```python
from build123d import *

# Parameters (mm, degrees)
ESTRUSIONE_ESTRUSIONE1_DEPTH = 10
SCHIZZO3_W                   = 8
SCHIZZO3_H                   = 6
TAGLIO_ESTRUSIONE2_DEPTH     = 60.371710435
TAGLIO_ESTRUSIONE3_DEPTH     = 60.371710435


with BuildPart() as part:
    # Schizzo1 → Estrusione-Estrusione1 (new body)
    with BuildSketch(Plane(origin=(0, 0, 0), x_dir=(1, 0, 0), z_dir=(0, 1, 0))):
        with BuildLine():
            Line((-25, 37.416573868), (-25, 30))
            Line((-25, 30), (25, 30))
            Line((25, 30), (25, 37.416573868))
            ThreePointArc((25, 37.416573868), (45, 0), (25, -37.416573868))
            Line((25, -37.416573868), (25, -30))
            Line((25, -30), (-25, -30))
            Line((-25, -30), (-25, -37.416573868))
            ThreePointArc((-25, -37.416573868), (-45, 0), (-25, 37.416573868))
        make_face()
    extrude(amount=ESTRUSIONE_ESTRUSIONE1_DEPTH)

    # Schizzo3 → Taglio-Estrusione2 (cut, through all)
    with BuildSketch(Plane(origin=(0, 10, 0), x_dir=(1, 0, 0), z_dir=(0, 1, 0))):
        with BuildLine():
            Line((-4, -3), (-4, 3))
            ThreePointArc((-4, 3), (-5, 0), (-4, -3))
        make_face()
        Rectangle(SCHIZZO3_W, SCHIZZO3_H)
        with BuildLine():
            ThreePointArc((5, 0), (4.74341649, 1.58113883), (4, 3))
            Line((4, 3), (4, -3))
            ThreePointArc((4, -3), (4.74341649, -1.58113883), (5, 0))
        make_face()
    extrude(amount=-TAGLIO_ESTRUSIONE2_DEPTH, mode=Mode.SUBTRACT)

    # Schizzo5 → Taglio-Estrusione3 (cut, through all)
    with BuildSketch(Plane(origin=(0, 10, 0), x_dir=(1, 0, 0), z_dir=(0, 1, 0))):
        Polygon((8, -25), (8, -28.5), (8, -30), (12, -30), (12, -27), (12, -25), (13.5, -25), (13.5, -21.5), (6.5, -21.5), (6.5, -25), align=None)
        Polygon((-13.5, 21.5), (-6.5, 21.5), (-6.5, 25), (-8, 25), (-8, 28.5), (-8, 30), (-12, 30), (-12, 28.5), (-12, 25), (-13.5, 25), align=None)
        Polygon((6.5, 21.5), (13.5, 21.5), (13.5, 25), (12, 25), (12, 27), (12, 30), (8, 30), (8, 28.5), (8, 25), (6.5, 25), align=None)
        Polygon((-8, -28.5), (-8, -25), (-6.5, -25), (-6.5, -21.5), (-13.5, -21.5), (-13.5, -25), (-12, -25), (-12, -28.5), (-12, -30), (-8, -30), align=None)
    extrude(amount=-TAGLIO_ESTRUSIONE3_DEPTH, mode=Mode.SUBTRACT)


solid = part.part
```
Input: part model. Units: mm. Frame: model coordinates. A direction names the side the tool comes from. Give positions to 0.01 mm unless a question says otherwise; leave off trailing zeros. Write each loop counter-clockwise with the first axis right and the second up, starting at its lowest first coordinate (ties: lowest second). Pieces come first, ordered by that corner, then holes. Notation, with made-up numbers: (6.25, -7.75) - (26.25, -7.75) arc R22 cw to (26.25, 11.25) - close; hole circle Ø2 at (68.25, -18.75). An arc over 180 degrees is marked (long way). Write item = value, one per line. Start each with the question number.
1) Draft query along Z for faces 5 (the face through (6.5, 5, 23)), 6 (the face through (10, 5, -21.5)), 7 (the face through (-8, 5, 28)), 8 (the face through (19, 5, 30)). Return one class per face: pulls with the +Z half, pulls with the -Z half, needs draft (parallel to the pull), parting line crosses it, or undercut.
2) Pin query (flat end, axial travel): pin 1 (1.6 mm diameter, centred on x = 13, y = 4.5, fed in from -Z); pin 2 (5.5 mm diameter, centred on x = -11, y = 3.5, fed in from +Z); pin 3 (4 mm diameter, centred on y = 4.5, z = 24, fed in from -X). Return the tip coordinate at first contact, or that it passes through.
3) Reachability of faces 1 (the face through (1, 10, 8)), 2 (the face through (-12, 5, 27)), 3 (the face through (-8, 5, -27)), 4 (the face through (-13.5, 5, 23)) from +Z, -Z, +X, -X, +Y, -Y: full face, straight path, thin tool, end or side. Return the list, or none.
4) Cut plane C-C (z = 11). Return loops of the section in (x, y), and give its area (3 significant figures).
5) Cut plane B-B (x = 22). Return loops of the section in (y, z), and give its area (3 significant figures).
6) Material intervals for L1, parallel to X at y = 1, z = -26.5; L2, parallel to X at y = 6.25, z = 28; L3, parallel to Z at x = -23.5, y = 2, sorted ascending. Write a range as [from, to].
7) Cut plane A-A (z = -26). Return loops of the section in (x, y), and give its area (3 significant figures).
Answers follow:
q1.face_5 = undercut
q1.face_6 = undercut
q1.face_7 = needs draft
q1.face_8 = pulls with the +Z half
q2.pin_1 = -30
q2.pin_2 = 30
q2.pin_3 = -39.26
q3.face_1 = +Z, -Z, +X, -X, +Y
q3.face_2 = +Z, +Y, -Y
q3.face_3 = -Z, +Y, -Y
q3.face_4 = +Y, -Y
q4.outline = (-43.63, 0) - (43.63, 0) - (43.63, 10) - (-43.63, 10) - close
q4.area = 873 mm^2
q5.outline = (0, -30) - (10, -30) - (10, 30) - (0, 30) - close
q5.area = 600 mm^2
q6.L1 = [-36.37, -12], [-8, 8], [12, 36.37]
q6.L2 = [-35.23, -12], [-8, 8], [12, 35.23]
q6.L3 = [-30, 30]
q7.outline = (-36.73, 0) - (-12, 0) - (-12, 10) - (-36.73, 10) - close; (-8, 0) - (8, 0) - (8, 10) - (-8, 10) - close; (12, 0) - (36.73, 0) - (36.73, 10) - (12, 10) - close
q7.area = 655 mm^2
